Geometry: final body of the model. Coordinates: model frame, mm. A direction names the side the tool comes from. Coordinates: 2 decimals unless noted, no trailing zeros. Loops run counter-clockwise (first coordinate to the right, second up) from the corner with the lowest first, then second, coordinate; pieces in that order, holes last. Notation, with made-up numbers: (11, -3.75) - (19, -3.75) arc R18 ccw to (19, 20.25) - close; hole circle Ø8 at (83.5, -28.5). An arc over 180 degrees is marked (long way). Answer in a Markdown table with one row per item.
from build123d import *
from OCP.BRepFilletAPI import BRepFilletAPI_MakeChamfer

# Parameters (mm, degrees)
SKETCH_1_R      = 0.66
EXTRUDE_START   = 4
SKETCH_3_R      = 2.8
EXTRUDE_1_DEPTH = 9
CHAMFER_1_SIZE  = 0.4
CHAMFER_1_SIZE2 = 0.145588094


with BuildPart() as part:
    # По траектории1: sweep along a path in Эскиз2
    with BuildLine(Plane.XY) as sweep_1_path:
        Line((0, 0), (0, 14.5))
        ThreePointArc((0, 14.5), (0.585786438, 15.914213562), (2, 16.5))
        Line((2, 16.5), (3, 16.5))
        ThreePointArc((3, 16.5), (4.414213562, 15.914213562), (5, 14.5))
        Line((5, 14.5), (5, 0))
    # Эскиз1 → По траектории1 (sweep)
    with BuildSketch(Plane(origin=(0, 0, 0), x_dir=(1, 0, 0), z_dir=(0, 1, 0))):
        Circle(SKETCH_1_R)
    sweep(path=sweep_1_path.line)

    # Эскиз3 → Бобышка-Вытянуть1 (add)
    with BuildSketch(Plane(origin=(0, 0, 0), x_dir=(1, 0, 0), z_dir=(0, 1, 0)).offset(EXTRUDE_START)):
        with Locations(Location((0, 0, 0), (0, 0, 270))):
            Circle(SKETCH_3_R)
    extrude(amount=EXTRUDE_1_DEPTH)

    # Фаска1: one chamfer whose edges measure the first distance from different faces: ONE call of the kernel's chamfer builder (chamfer() names one face for all edges)
    chamfer_1_edges_1 = [part.edges().sort_by_distance(p)[0] for p in [
        (-0.66, 0, 0),
    ]]
    chamfer_1_side_1 = [part.faces().sort_by_distance(p)[0] for p in [
        (-0.66, 2, 0),
    ]]
    chamfer_1_edges_2 = [part.edges().sort_by_distance(p)[0] for p in [
        (5.66, 0, 0),
    ]]
    chamfer_1_side_2 = [part.faces().sort_by_distance(p)[0] for p in [
        (5.66, 7.25, 0),
    ]]
    chamfer_1 = BRepFilletAPI_MakeChamfer(part.part.solid().wrapped)
    for e in chamfer_1_edges_1:
        chamfer_1.Add(CHAMFER_1_SIZE, CHAMFER_1_SIZE2, e.wrapped, chamfer_1_side_1[0].wrapped)  # the first distance lies on this face
    for e in chamfer_1_edges_2:
        chamfer_1.Add(CHAMFER_1_SIZE, CHAMFER_1_SIZE2, e.wrapped, chamfer_1_side_2[0].wrapped)  # the first distance lies on this face
    add(Compound.cast(chamfer_1.Shape()), mode=Mode.REPLACE)


solid = part.part
(1) Cut plane C-C on y = 2.75. Output: boundary loops of the cut face in (x, z), then the cut area to 3 significant figures.
Verdict:
| item | result |
|---|---|
| outline | circle Ø1.32 at (0, 0); circle Ø1.32 at (5, 0) |
| area | 2.74 mm² |
(2) Ray query, probe 1 along Y at (x, z) = (-1.75, -2); probe 2 along X at (y, z) = (6.5, 0.15); probe 3 along Z at (x, y) = (5, 1.5). Return the intervals inside material, ascending.
Verdict:
| item | result |
|---|---|
| probe 1 | y = 4 to 13 |
| probe 2 | x = -2.8 to 2.8, 4.36 to 5.64 |
| probe 3 | z = -0.66 to 0.66 |
(3) Access query for faces 1 (the face through (0, 0, 0)), 2 (the face through (4.37, 7.35, -0.2)), 3 (the face through (-0.143, 13.76, 0.644)). Directions: +Z, -Z, +X, -X, +Y, -Y. A direction counts if a zero-diameter tool reaches every point of the face in a straight line with its end or side. Return the directions, or none.
Verdict:
| item | result |
|---|---|
| face 1 | +Z, -Z, +X, -X, -Y |
| face 2 | -Y |
| face 3 | none |
(4) Cut plane A-A on y = 8.25. Output: boundary loops of the cut face in (x, z), then the cut area to 3 significant figures.
Verdict:
| item | result |
|---|---|
| outline | circle Ø5.6 at (0, 0); circle Ø1.32 at (5, 0) |
| area | 26.0 mm² |
(5) First-contact query: pin 1 Ø1 at (y, z) = (15.5, 0) entering from +X; pin 2 Ø1 at (x, z) = (4, 1.5) entering from -Y; pin 3 Ø1.5 at (x, z) = (0, 1) entering from +Y. Flat tips, straight axial feed; report the tip coordinate or a pass-through.
Verdict:
| item | result |
|---|---|
| pin 1 | stops at x = 5.61 |
| pin 2 | passes through |
| pin 3 | stops at y = 16.49 |
(6) Pull-direction query (X, two-part tool) for faces 4 (the face through (2.51, 17.16, -0.03)), 5 (the face through (5, 0, 0)); classes: pulls with the +X half, pulls with the -X half, needs draft (parallel to the pull), parting line crosses it, or undercut.
Verdict:
| item | result |
|---|---|
| face 4 | undercut |
| face 5 | needs draft |
(7) Cut plane D-D on x = -1.75. Output: boundary loops of the cut face in (y, z).
Verdict:
| item | result |
|---|---|
| outline | (4, -2.19) - (13, -2.19) - (13, 2.19) - (4, 2.19) - close |
(8) Cut plane B-B on z = 0. Output: boundary loops of the cut face in (x, y).
Verdict:
| item | result |
|---|---|
| outline | (-2.8, 4) - (-0.66, 4) - (-0.66, 0.4) - (-0.51, 0) - (0.51, 0) - (0.66, 0.4) - (0.66, 4) - (2.8, 4) - (2.8, 13) - (0.66, 13) - (0.66, 14.5) arc R1.34 cw to (2, 15.84) - (3, 15.84) arc R1.34 cw to (4.34, 14.5) - (4.34, 0.4) - (4.49, 0) - (5.51, 0) - (5.66, 0.4) - (5.66, 14.5) arc R2.66 ccw to (3, 17.16) - (2, 17.16) arc R2.66 ccw to (-0.66, 14.5) - (-0.66, 13) - (-2.8, 13) - close |
